Geometry: final body of the model. Coordinates: model frame, mm. A direction names the side the tool comes from. Give positions to 0.01 mm unless a question says otherwise; leave off trailing zeros. Order: outer loops, then holes, each group sorted by start corner. A loop starts at its lowest first (then second) coordinate and runs counter-clockwise, first axis right, second up. Notation, with made-up numbers: (27.5, 81) - (73.5, 81) arc R14 cw to (73.5, 89) - close; hole circle Ø11 at (-26, 70.25). An arc over 180 degrees is marked (long way). Put each result on its own line as item: value. Start each with the question number.
1. Section A-A on y = 7.5. Return the cut outline in (x, z), plus the area to 3 significant figures.
2. First-contact query: P1, Ø0.9, axis at y = 3, z = -20.5, coming from the +X side; P2, Ø3, axis at y = 8, z = 18, coming from the -X side; P3, Ø5, axis at y = 7.5, z = 16.5, coming from the +X side; P4, Ø4, axis at x = 10, y = 4, coming from the +Z side. Flat tips, straight axial feed; report the tip coordinate or a pass-through.
3. Mould query, pull axis Y, two halves, no side actions, for faces 5 (the cylindrical face through (-0.651, 2.543, 38.895)), 6 (the flat face through (0, 7, 11.5)), 7 (the flat face through (2.5, 2, -21)), 8 (the flat face through (-13, 11.5, 19)). Classes: pulls with the +Y half, pulls with the -Y half, needs draft (parallel to the pull), parting line crosses it, or undercut.
4. Ray query, line 1 along Y through (x, z) = (0, 36); line 2 along X through (y, z) = (7.75, 34); line 3 along Y through (x, z) = (-12.75, -14). Return the intervals inside material, ascending. Write a range as from..to.
5. Set-up query: faces 1 (the cylindrical face through (-11.978, 11.246, 18.515)), 2 (the cylindrical face through (-0.92, 3.35, 39.11)), 3 (the flat face through (0, 1.618, -21)), 4 (the flat face through (7.5, 7, 17)). Return all of +Z, -Z, +X, -X, +Y, -Y with unobstructed straight access to the full face (end or side cutting, diameter ignored); none if empty.
6. Section C-C on x = -3.5. Return the cut outline in (y, z), plus the area to 3 significant figures.
7. Section D-D on z = 8.5. Return the cut outline in (x, y), plus the area to 3 significant figures.
8. Section B-B on z = 27. Return the cut outline in (x, y), plus the area to 3 significant figures.
Autodesk Inventor part; units mm, degrees
ref_plane "YZ Plane" through (0, 0, 0) normal (1, 0, 0) x (0, 1, 0)
ref_plane "XZ Plane" through (0, 0, 0) normal (0, 1, 0) x (-1, 0, 0)
ref_plane "XY Plane" through (0, 0, 0) normal (0, 0, 1) x (1, 0, 0)
sketch "Sketch1" plane through (0, 0, 0) normal (0, 1, 0) x (-1, 0, 0)
  line L0 (-15, 21.5) -> (-15, -21.5)
  line L1 (-15, -21.5) -> (15, -21.5)
  line L2 (15, -21.5) -> (15, 21.5)
  line L3 (15, 21.5) -> (-15, 21.5)
  line L4 (-15, 21.5) -> (15, -21.5) construction
  line L5 (-15, -21.5) -> (15, 21.5) construction
  point P0 (0, 0)
  dimension "d0" = 43
  dimension "d1" = 30
extrude "Extrusion1" add sketch "Sketch1" along normal blind 1
sketch "Sketch2" plane through (0, 1, 0) normal (0, 1, 0) x (1, 0, 0)
  line L0 (4.25, 16.6043) -> (4.25, 21.5)
  line L1 (4.25, 21.5) -> (-4.25, 21.5)
  line L2 (-4.25, 21.5) -> (-4.25, 16.6043)
  line L3 (-4.25, 16.6043) -> (4.25, 16.6043)
  line L4 (4.25, 16.6043) -> (-4.25, 21.5) construction
  line L5 (4.25, 21.5) -> (-4.25, 16.6043) construction
  line L6 (-15, 21.5) -> (-15, -21.5) construction
  line L7 (-15, 0) -> (-12, 0) construction
  line L8 (-12, 0) -> (-12, -1.5) construction
  line L9 (-12, -1.5) -> (-7, -1.5) construction
  line L10 (-7, -1.5) -> (-7, 1.5) construction
  line L11 (-12, -1.5) -> (-7, -1.5)
  line L12 (-7, -1.5) -> (-7, 1.5)
  line L13 (-7, 1.5) -> (-12, 1.5)
  line L14 (-12, 1.5) -> (-12, -1.5)
  line L15 (15, -21.5) -> (15, 21.5)
  line L16 (15, 0) -> (5, 0) construction
  line L17 (5, 0) -> (5, -1.5)
  line L18 (5, -1.5) -> (0, -1.5)
  line L19 (0, -1.5) -> (0, 1.5)
  line L20 (0, 1.5) -> (5, 1.5)
  line L21 (5, 1.5) -> (5, 0)
  line L22 (0, -21.5) -> (7.5, -21.5)
  line L23 (-15, -21.5) -> (15, -21.5)
  line L24 (7.5, -21.5) -> (7.5, -11.5)
  line L25 (7.5, -11.5) -> (-7.5, -11.5)
  line L26 (-7.5, -11.5) -> (-7.5, -21.5)
  line L27 (-7.5, -21.5) -> (7.5, -21.5)
  line L28 (-7.5, -11.5) -> (-8.5, -11.5) construction
  line L29 (-8.5, -11.5) -> (-13.5, -11.5)
  line L30 (-13.5, -11.5) -> (-13.5, -20.6777)
  line L31 (-13.5, -20.6777) -> (-8.5, -20.6777)
  line L32 (-8.5, -20.6777) -> (-8.5, -11.5)
  point P0 (0, 0)
  point P1 (0, 19.0521)
  dimension "d4" = 8.5
  dimension "d5" = 3
  dimension "d6" = 1.5
  dimension "d7" = 5
  dimension "d8" = 3
  dimension "d9" = 10
  dimension "d10" = 1.5
  dimension "d11" = 5
  dimension "d12" = 3
  dimension "d13" = 5
  dimension "d14" = 7.5
  dimension "d15" = 10
  dimension "d16" = 15
  dimension "d17" = 1
extrude "Extrusion2" add sketch "Sketch2" along normal blind 1 contours L14 L13 L12 L11 | L17 L18 L19 L20 L21
extrude "Extrusion3" add sketch "Sketch2" along normal blind 3 contours L3 L2 L1 L0
extrude "Extrusion4" add sketch "Sketch2" along normal blind 13 contours L23 L26 L25 L24 L22
extrude "Extrusion5" add sketch "Sketch2" along normal blind 10 contours L32 L31 L30 L29
sketch "Sketch3" plane through (0, 11, 0) normal (0, 1, 0) x (1, 0, 0)
  circle A0 centre (-12.491, -19.5006) radius 1.111
  point P0 (0, 0)
extrude "Extrusion6" add sketch "Sketch3" along normal blind 0.5
sketch "Sketch4" plane through (0, 14, 0) normal (0, 1, 0) x (1, 0, 0)
  line L0 (7.5, -11.5) -> (7.5, -21.5) construction
  line L1 (7.5, -11.5) -> (-7.5, -11.5) construction
  line L2 (7.5, -21.5) -> (-7.5, -11.5) construction
  line L3 (-7.5, -11.5) -> (-7.5, -21.5) construction
  line L4 (-15, -21.5) -> (15, -21.5) construction
  line L5 (-7.5, -21.5) -> (7.5, -11.5) construction
  line L6 (5.8773, -20.4182) -> (-5.8773, -20.4182) construction
  line L7 (-5.8773, -20.4182) -> (-5.8773, -14.4182) construction
  line L8 (-5.8773, -14.4182) -> (5.8773, -14.4182) construction
  line L9 (5.8773, -14.4182) -> (5.8773, -20.4182) construction
  line L10 (5.8773, -20.4182) -> (-5.8773, -20.4182)
  line L11 (-5.8773, -20.4182) -> (-5.8773, -14.4182)
  line L12 (-5.8773, -14.4182) -> (5.8773, -14.4182)
  line L13 (5.8773, -14.4182) -> (5.8773, -20.4182)
  point P0 (0, 0)
  dimension "d28" = 6
extrude "Extrusion7" cut sketch "Sketch4" against normal blind 2
sketch "Sketch5" plane through (15, 0, -21.5) normal (0, 0, -1) x (-1, 0, 0)
  line L0 (10.75, 1) -> (10.75, 4)
  line L1 (19.25, 1) -> (19.25, 4)
  line L2 (10.75, 1) -> (19.25, 1)
  line L3 (10.75, 1) -> (19.25, 4) construction
  line L4 (19.25, 1) -> (10.75, 4) construction
  line L5 (12.5, 1.6176) -> (12.5, 3.3824)
  line L6 (12.5, 1.6176) -> (17.5, 1.6176)
  line L7 (17.5, 1.6176) -> (17.5, 3.3824)
  line L8 (17.5, 3.3824) -> (12.5, 3.3824)
  point P0 (15, 0)
extrude "Extrusion8" cut sketch "Sketch5" against normal blind 2
sketch "Sketch6" plane through (-15, 0, 21.5) normal (0, 0, 1) x (1, 0, 0)
  line L0 (0, 0) -> (30, 0)
  line L1 (30, 0) -> (30, 1)
  line L2 (22.5, 1) -> (30, 1)
  line L3 (22.5, 1) -> (22.5, 14)
  line L4 (7.5, 14) -> (22.5, 14)
  line L5 (7.5, 1) -> (7.5, 14)
  line L6 (0, 1) -> (7.5, 1)
  line L7 (0, 0) -> (0, 1)
  circle A0 centre (15, 7.5) radius 6.5
  point P0 (15, 0)
extrude "Extrusion9" add sketch "Sketch6" along normal blind 10 contours A0
sketch "Sketch7" plane through (0, 7.5, 31.5) normal (0, 0, 1) x (1, 0, 0)
  circle A0 centre (0, 0) radius 5
  point P0 (0, -7.5)
  dimension "d35" = 10
extrude "Extrusion10" add sketch "Sketch7" along normal blind 15
thread "Thread1"
sketch "Sketch8" plane through (0, 7.5, 46.5) normal (0, 0, 1) x (1, 0, 0)
  circle A0 centre (0, 0) radius 5
  circle A1 centre (0, 0) radius 4.25
  point P0 (0, -7.5)
  dimension "d40" = 0.75
extrude "Extrusion11" cut sketch "Sketch8" against normal blind 15 contours A1
properties part number "Ph Reader"
Resolved:
1. outline: (-13.5, 11.5) - (-8.5, 11.5) - (-8.5, 20.68) - (-13.5, 20.68) - close; (-7.5, 11.5) - (7.5, 11.5) - (7.5, 21.5) - (6.5, 21.5) - (6.5, 31.5) - (5, 31.5) - (5, 46.5) - (4.25, 46.5) - (4.25, 31.5) - (-4.25, 31.5) - (-4.25, 46.5) - (-5, 46.5) - (-5, 31.5) - (-6.5, 31.5) - (-6.5, 21.5) - (-7.5, 21.5) - close
1. area: 348 mm^2
2. P1: x = 4.25
2. P2: x = -13.5
2. P3: x = 7.5
2. P4: through
3. face 5: parting line crosses it
3. face 6: needs draft
3. face 7: undercut
3. face 8: pulls with the +Y half
4. line 1: 2.5..3.25, 11.75..12.5
4. line 2: -4.99..-4.24, 4.24..4.99
4. line 3: 0..1
5. face 1: +Y
5. face 2: +Z
5. face 3: -Z
5. face 4: +Z, -Z, +X, +Y
6. outline: (0, -21.5) - (4, -21.5) - (4, -16.6) - (1, -16.6) - (1, 11.5) - (14, 11.5) - (14, 14.42) - (12, 14.42) - (12, 20.42) - (14, 20.42) - (14, 21.5) - (12.98, 21.5) - (12.98, 31.5) - (11.07, 31.5) - (11.07, 46.5) - (9.91, 46.5) - (9.91, 31.5) - (5.09, 31.5) - (5.09, 46.5) - (3.93, 46.5) - (3.93, 31.5) - (2.02, 31.5) - (2.02, 21.5) - (0, 21.5) - close
6. area: 320 mm^2
7. outline: (-15, 0) - (15, 0) - (15, 1) - (-15, 1) - close
7. area: 30.0 mm^2
8. outline: circle Ø13 at (0, 7.5)
8. area: 133 mm^2
